Read the model definition and answer for the solid it produces. Units are mm, in the model's axes. Face numbers are marked on the shaded views. A direction names the side the tool comes from. Round coordinates to 2 decimals unless told otherwise and drop trailing zeros. Write each loop counter-clockwise with the first axis right and the second up, starting at its lowest first coordinate (ties: lowest second). Pieces come first, ordered by that corner, then holes. Notation, with made-up numbers: (-31.75, 13.5) -> (-22.75, 13.5) arc R20 cw to (-22.75, 26.5) -> close; hole circle Ø7 at (9.25, -30). An arc over 180 degrees is marked (long way). Return JSON: item names as keys, results as strings. Group by question number.
(1) A cutting plane is placed at C-C on z = 0. Give the vertices of the cut face in (x, y).
(2) A cutting plane is placed at A-A on y = 0.2. Give the vertices of the cut face in (x, z), then the cut area to 3 significant figures.
(3) Given pin 1 (1.5 mm diameter, centred on y = 0.5, z = -2, fed in from +X), flat-ended and moving along its own axis, determine where the tip first touches the part or whether it passes through.
(4) A cutting plane is placed at D-D on y = 1.05. Give the vertices of the cut face in (x, z), then the cut area to 3 significant figures.
(5) A cutting plane is placed at B-B on x = 0. Give the vertices of the cut face in (y, z), then the cut area to 3 significant figures.
(6) The mould has two halves that part along Z. Classify the marked faces 3 and 4: released by +Z, released by -Z, zero draft, split by the parting line, or undercut.
(7) For the marked faces 1 and 2, determine the directions among +Z, -Z, +X, -X, +Y, -Y from which every point of the face is accessible in a straight line to the end or side of a thin tool.
(8) Straight lines are drawn through the part: line 1 (Z direction, x = 0, y = 3.6); line 2 (Z direction, x = 0, y = 1.1); line 3 (Y direction, x = -3.75, z = 2.5). For each, find the intervals that lie inside material, in ascending order.
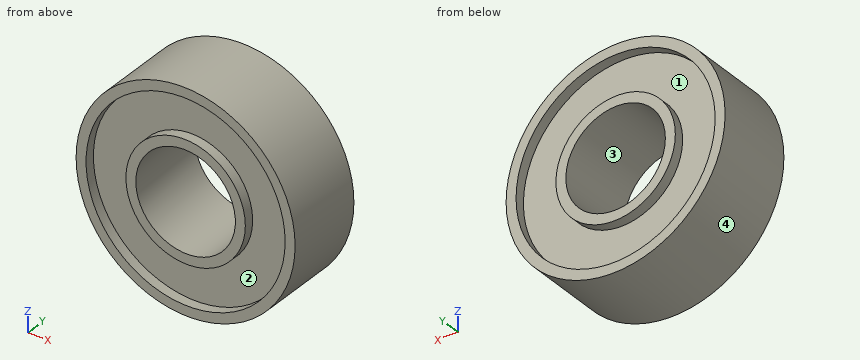
Autodesk Inventor part; units mm, degrees
ref_plane "YZ Plane" through (0, 0, 0) normal (1, 0, 0) x (0, 1, 0)
ref_plane "XZ Plane" through (0, 0, 0) normal (0, 1, 0) x (-1, 0, 0)
ref_plane "XY Plane" through (0, 0, 0) normal (0, 0, 1) x (1, 0, 0)
sketch "Sketch1" plane through (0, 0, 0) normal (0, 1, 0) x (-1, 0, 0)
  circle A0 centre (0, 0) radius 5.5
  circle A1 centre (0, 0) radius 2.5
  dimension "d0" = 11
  dimension "d1" = 5
extrude "Extrusion1" add sketch "Sketch1" along normal blind 4
sketch "Sketch2" plane through (0, 4, 0) normal (0, 1, 0) x (1, 0, 0)
  circle A0 centre (0, 0) radius 5.5
  circle A1 centre (0, 0) radius 2.5
  circle A2 centre (0, 0) radius 3
  circle A3 centre (0, 0) radius 5
  dimension "d4" = 0.5
  dimension "d5" = 0.5
extrude "Extrusion2" cut sketch "Sketch2" against normal blind 0.5 contours A3
sketch "Sketch3" plane through (0, 0, 0) normal (0, -1, 0) x (1, 0, 0)
  circle A0 centre (0, 0) radius 5.5
  circle A1 centre (0, 0) radius 2.5
  circle A2 centre (0, 0) radius 5
  circle A3 centre (0, 0) radius 3
extrude "Extrusion3" cut sketch "Sketch3" against normal blind 0.5 contours A2
properties part number "Bearing_5x11x4"
Checks:
{
 "1": {"outline": "(-5.5, 0) -> (-5, 0) -> (-5, 0.5) -> (-3, 0.5) -> (-3, 0) -> (-2.5, 0) -> (-2.5, 4) -> (-3, 4) -> (-3, 3.5) -> (-5, 3.5) -> (-5, 4) -> (-5.5, 4) -> close; (2.5, 0) -> (3, 0) -> (3, 0.5) -> (5, 0.5) -> (5, 0) -> (5.5, 0) -> (5.5, 4) -> (5, 4) -> (5, 3.5) -> (3, 3.5) -> (3, 4) -> (2.5, 4) -> close"},
 "2": {"outline": "circle Ø11 at (0, 0); circle Ø6 at (0, 0); hole circle Ø10 at (0, 0); hole circle Ø5 at (0, 0)", "area": "25.1 mm^2"},
 "3": {"pin 1": "stops at x = 5.36"},
 "4": {"outline": "circle Ø11 at (0, 0); hole circle Ø5 at (0, 0)", "area": "75.4 mm^2"},
 "5": {"outline": "(0, -5.5) -> (4, -5.5) -> (4, -5) -> (3.5, -5) -> (3.5, -3) -> (4, -3) -> (4, -2.5) -> (0, -2.5) -> (0, -3) -> (0.5, -3) -> (0.5, -5) -> (0, -5) -> close; (0, 2.5) -> (4, 2.5) -> (4, 3) -> (3.5, 3) -> (3.5, 5) -> (4, 5) -> (4, 5.5) -> (0, 5.5) -> (0, 5) -> (0.5, 5) -> (0.5, 3) -> (0, 3) -> close", "area": "20.0 mm^2"},
 "6": {"face 3": "undercut", "face 4": "split by the parting line"},
 "7": {"face 1": "+Y", "face 2": "-Y"},
 "8": {"line 1": "z = -5.5 to -5, -3 to -2.5, 2.5 to 3, 5 to 5.5", "line 2": "z = -5.5 to -2.5, 2.5 to 5.5", "line 3": "y = 0.5 to 3.5"}
}
